```python
from build123d import *

# Parameters (mm, degrees)
F0_DEPTH     = 70
F1_W         = 75
F1_H         = 15
F4_DEPTH     = 2
F2_T1_DEPTH  = 11
F2_T3_DEPTH  = 73
F2_T5_DEPTH  = 67
F2_T7_DEPTH  = 71
F2_S11_W     = 2.04
F2_S11_H     = 2.04
F2_T12_DEPTH = 2.04
F2_S17_W     = 2.04
F2_S17_H     = 2.04
F2_T18_DEPTH = 2.04
F2_S23_W     = 2.04
F2_S23_H     = 2.04
F2_T24_DEPTH = 2.04
F2_S29_W     = 2.04
F2_S29_H     = 2.04
F2_T30_DEPTH = 2.04
F2_T37_DEPTH = 73
F2_T42_DEPTH = 72
F2_T50_DEPTH = 72
F2_T55_DEPTH = 73
F2_T62_DEPTH = 16
F2_T67_DEPTH = 16


# Not quite as in the source:
# - a fillet or chamfer that OpenCascade refuses, or shapes differently, is made with other operations: its cross-section is extruded or revolved along the edge and cut away or added
# - a feature names something its author has since deleted; it is built from what else it names


with BuildPart() as f0:
    # F3 (on Top) → F0 (new body)
    with BuildSketch(Plane.XY):
        Polygon((-37.5, 15), (-37.5, 0), (37.5, 0), (37.5, 15), (33.5, 15), (33.5, 13), (35.5, 13), (35.5, 2), (-35.5, 2), (-35.5, 13), (-33.5, 13), (-33.5, 15), align=None)
    extrude(amount=F0_DEPTH)

    # F1 (on face) → F4 (join)
    with BuildSketch(Plane(origin=(0, 0, 0), x_dir=(1, 0, 0), z_dir=(0, 0, -1))):
        with Locations((0, -7.5)):
            Rectangle(F1_W, F1_H)
    extrude(amount=-F4_DEPTH)

    # F2: fillet of radius 2 on 13 edges, made by hand

    # F2_s2 → F2_t1 (cut)
    with BuildSketch(Plane.XZ.offset(-13)):
        with BuildLine():
            ThreePointArc((37.5, 2), (36.9142135624, 0.5857864376), (35.5, 0))
            Line((35.5, 0), (37.5, 0))
            Line((37.5, 0), (37.5, 2))
        make_face()
        with BuildLine():
            ThreePointArc((-37.5, 2), (-36.9142135624, 0.5857864376), (-35.5, 0))
            Line((-35.5, 0), (-37.5, 0))
            Line((-37.5, 0), (-37.5, 2))
        make_face()
    extrude(amount=F2_T1_DEPTH, mode=Mode.SUBTRACT)

    # F2_s4 → F2_t3 (cut)
    with BuildSketch(Plane.XY.offset(2)):
        with BuildLine():
            ThreePointArc((-37.5, 2), (-36.9142135624, 0.5857864376), (-35.5, 0))
            Line((-35.5, 0), (-37.5, 0))
            Line((-37.5, 0), (-37.5, 2))
        make_face()
        with BuildLine():
            ThreePointArc((35.5, 0), (36.9142135624, 0.5857864376), (37.5, 2))
            Line((37.5, 2), (37.5, 0))
            Line((37.5, 0), (35.5, 0))
        make_face()
        with BuildLine():
            ThreePointArc((-37.5, 13), (-36.9142135624, 14.4142135624), (-35.5, 15))
            Line((-35.5, 15), (-37.5, 15))
            Line((-37.5, 15), (-37.5, 13))
        make_face()
        with BuildLine():
            ThreePointArc((37.5, 13), (36.9142135624, 14.4142135624), (35.5, 15))
            Line((35.5, 15), (37.5, 15))
            Line((37.5, 15), (37.5, 13))
        make_face()
        with BuildLine():
            ThreePointArc((-33.5, 13), (-34.0857864376, 14.4142135624), (-35.5, 15))
            Line((-35.5, 15), (-33.5, 15))
            Line((-33.5, 15), (-33.5, 13))
        make_face()
        with BuildLine():
            ThreePointArc((33.5, 13), (34.0857864376, 14.4142135624), (35.5, 15))
            Line((35.5, 15), (33.5, 15))
            Line((33.5, 15), (33.5, 13))
        make_face()
    extrude(amount=F2_T3_DEPTH, mode=Mode.SUBTRACT)

    # F2_s6 → F2_t5 (cut)
    with BuildSketch(Plane.YZ.offset(-33.5)):
        with BuildLine():
            ThreePointArc((13, 2), (14.4142135624, 1.4142135624), (15, 0))
            Line((15, 0), (15, 2))
            Line((15, 2), (13, 2))
        make_face()
    extrude(amount=F2_T5_DEPTH, mode=Mode.SUBTRACT)

    # F2_s8 → F2_t7 (cut)
    with BuildSketch(Plane.YZ.offset(-35.5)):
        with BuildLine():
            ThreePointArc((0, 2), (0.5857864376, 0.5857864376), (2, 0))
            Line((2, 0), (0, 0))
            Line((0, 0), (0, 2))
        make_face()
        with BuildLine():
            ThreePointArc((15, 2), (14.4142135624, 0.5857864376), (13, 0))
            Line((13, 0), (15, 0))
            Line((15, 0), (15, 2))
        make_face()
    extrude(amount=F2_T7_DEPTH, mode=Mode.SUBTRACT)


with BuildPart() as f2_tool10:
    # F2_s11 → F2_t12 (new body)
    with BuildSketch(Plane.XZ.offset(-2)):
        with Locations((36.52, 0.98)):
            Rectangle(F2_S11_W, F2_S11_H)
    extrude(amount=F2_T12_DEPTH)

    # F2_s13 → F2_t14 (revolve, cut)
    with BuildSketch(Plane(origin=(35.5, 2, 2), x_dir=(-0.7071067812, 0, 0.7071067812), z_dir=(0.7071067812, 0, 0.7071067812))):
        with BuildLine():
            ThreePointArc((0, -2), (2, 0), (0, 2))
            Line((0, 2), (0, -2))
        make_face()
    revolve(axis=Axis((35.5, 2, 2), (0, -1, 0)), mode=Mode.SUBTRACT)


with BuildPart() as f0_1:
    add(f0.part)

    # F2_t9: cut F2_tool10
    add(f2_tool10.part, mode=Mode.SUBTRACT)


with BuildPart() as f2_tool16:
    # F2_s17 → F2_t18 (new body)
    with BuildSketch(Plane.YZ.offset(35.5)):
        with Locations((14.02, 0.98)):
            Rectangle(F2_S17_W, F2_S17_H)
    extrude(amount=F2_T18_DEPTH)

    # F2_s19 → F2_t20 (revolve, cut)
    with BuildSketch(Plane(origin=(35.5, 13, 2), x_dir=(0, -0.7071067812, 0.7071067812), z_dir=(0, 0.7071067812, 0.7071067812))):
        with BuildLine():
            ThreePointArc((0, -2), (2, 0), (0, 2))
            Line((0, 2), (0, -2))
        make_face()
    revolve(axis=Axis((35.5, 13, 2), (1, 0, 0)), mode=Mode.SUBTRACT)


with BuildPart() as f0_2:
    add(f0_1.part)

    # F2_t15: cut F2_tool16
    add(f2_tool16.part, mode=Mode.SUBTRACT)


with BuildPart() as f2_tool22:
    # F2_s23 → F2_t24 (new body)
    with BuildSketch(Plane.YZ.offset(-35.5)):
        with Locations((14.02, 0.98)):
            Rectangle(F2_S23_W, F2_S23_H)
    extrude(amount=-F2_T24_DEPTH)

    # F2_s25 → F2_t26 (revolve, cut)
    with BuildSketch(Plane(origin=(-35.5, 13, 2), x_dir=(0, -0.7071067812, 0.7071067812), z_dir=(0, -0.7071067812, -0.7071067812))):
        with BuildLine():
            ThreePointArc((0, -2), (2, 0), (0, 2))
            Line((0, 2), (0, -2))
        make_face()
    revolve(axis=Axis((-35.5, 13, 2), (-1, 0, 0)), mode=Mode.SUBTRACT)


with BuildPart() as f0_3:
    add(f0_2.part)

    # F2_t21: cut F2_tool22
    add(f2_tool22.part, mode=Mode.SUBTRACT)


with BuildPart() as f2_tool28:
    # F2_s29 → F2_t30 (new body)
    with BuildSketch(Plane.YZ.offset(-35.5)):
        with Locations((0.98, 0.98)):
            Rectangle(F2_S29_W, F2_S29_H)
    extrude(amount=-F2_T30_DEPTH)

    # F2_s31 → F2_t32 (revolve, cut)
    with BuildSketch(Plane(origin=(-35.5, 2, 2), x_dir=(0, 0.7071067812, 0.7071067812), z_dir=(0, -0.7071067812, 0.7071067812))):
        with BuildLine():
            ThreePointArc((0, -2), (2, 0), (0, 2))
            Line((0, 2), (0, -2))
        make_face()
    revolve(axis=Axis((-35.5, 2, 2), (-1, 0, 0)), mode=Mode.SUBTRACT)


with BuildPart() as f0_4:
    add(f0_3.part)

    # F2_t27: cut F2_tool28
    add(f2_tool28.part, mode=Mode.SUBTRACT)


with BuildPart() as f2_tool35:
    # F2_s36 → F2_t37 (new body)
    with BuildSketch(Plane.XY.offset(-3)):
        with BuildLine():
            ThreePointArc((-33.5, 13), (-34.0857864376, 14.4142135624), (-35.5, 15))
            Line((-35.5, 15), (-33.5, 15))
            Line((-33.5, 15), (-33.5, 13))
        make_face()
    extrude(amount=F2_T37_DEPTH)

    split(bisect_by=Plane.XY.offset(2), keep=Keep.BOTTOM)

    split(bisect_by=Plane.XY, keep=Keep.TOP)


with BuildPart() as f2_tool40:
    # F2_s41 → F2_t42 (new body)
    with BuildSketch(Plane.YZ.offset(-38.5)):
        with BuildLine():
            ThreePointArc((13, 2), (14.4142135624, 1.4142135624), (15, 0))
            Line((15, 0), (15, 2))
            Line((15, 2), (13, 2))
        make_face()
    extrude(amount=F2_T42_DEPTH)

    split(bisect_by=Plane.YZ.offset(-33.5), keep=Keep.BOTTOM)

    split(bisect_by=Plane.YZ.offset(-35.5), keep=Keep.TOP)


with BuildPart() as f2_tool35_1:
    add(f2_tool35.part)

    # F2_t45: intersect F2_tool40
    add(f2_tool40.part, mode=Mode.INTERSECT)


with BuildPart() as f0_5:
    add(f0_4.part)

    # F2_t33: cut F2_tool35
    add(f2_tool35_1.part, mode=Mode.SUBTRACT)


with BuildPart() as f2_tool48:
    # F2_s49 → F2_t50 (new body)
    with BuildSketch(Plane.YZ.offset(-33.5)):
        with BuildLine():
            ThreePointArc((13, 2), (14.4142135624, 1.4142135624), (15, 0))
            Line((15, 0), (15, 2))
            Line((15, 2), (13, 2))
        make_face()
    extrude(amount=F2_T50_DEPTH)

    split(bisect_by=Plane.YZ.offset(35.5), keep=Keep.BOTTOM)

    split(bisect_by=Plane.YZ.offset(33.5), keep=Keep.TOP)


with BuildPart() as f2_tool53:
    # F2_s54 → F2_t55 (new body)
    with BuildSketch(Plane.XY.offset(-3)):
        with BuildLine():
            ThreePointArc((33.5, 13), (34.0857864376, 14.4142135624), (35.5, 15))
            Line((35.5, 15), (33.5, 15))
            Line((33.5, 15), (33.5, 13))
        make_face()
    extrude(amount=F2_T55_DEPTH)

    split(bisect_by=Plane.XY.offset(2), keep=Keep.BOTTOM)

    split(bisect_by=Plane.XY, keep=Keep.TOP)


with BuildPart() as f2_tool48_1:
    add(f2_tool48.part)

    # F2_t58: intersect F2_tool53
    add(f2_tool53.part, mode=Mode.INTERSECT)


with BuildPart() as f0_6:
    add(f0_5.part)

    # F2_t46: cut F2_tool48
    add(f2_tool48_1.part, mode=Mode.SUBTRACT)


with BuildPart() as f2_tool60:
    # F2_s61 → F2_t62 (new body)
    with BuildSketch(Plane.XZ.offset(3)):
        with BuildLine():
            ThreePointArc((35.5, 4), (34.9142135624, 2.5857864376), (33.5, 2))
            Line((33.5, 2), (35.5, 2))
            Line((35.5, 2), (35.5, 4))
        make_face()
    extrude(amount=-F2_T62_DEPTH)

    split(bisect_by=Plane.XZ, keep=Keep.BOTTOM)


with BuildPart() as f0_7:
    add(f0_6.part)

    # F2_t59: union F2_tool60
    add(f2_tool60.part)


with BuildPart() as f2_tool65:
    # F2_s66 → F2_t67 (new body)
    with BuildSketch(Plane.XZ.offset(-13)):
        with BuildLine():
            ThreePointArc((-35.5, 4), (-34.9142135624, 2.5857864376), (-33.5, 2))
            Line((-33.5, 2), (-35.5, 2))
            Line((-35.5, 2), (-35.5, 4))
        make_face()
    extrude(amount=F2_T67_DEPTH)

    split(bisect_by=Plane.XZ, keep=Keep.BOTTOM)


with BuildPart() as f0_8:
    add(f0_7.part)

    # F2_t64: union F2_tool65
    add(f2_tool65.part)


solid = f0_8.part
```
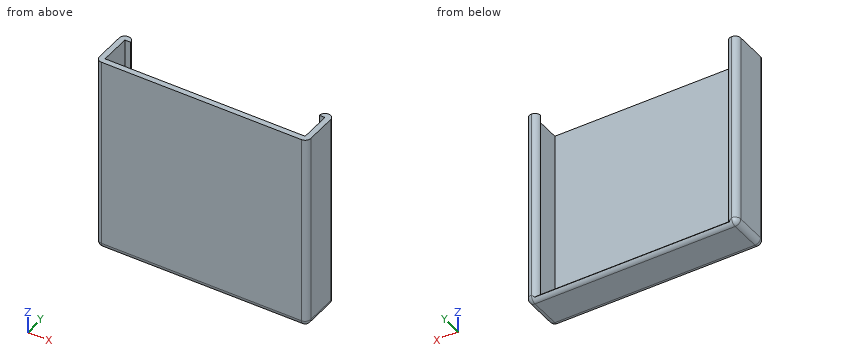
Design review of the part built by this model. Coordinates are the model's own, in mm. Coordinates: 2 decimals unless noted, no trailing zeros. Loops run counter-clockwise (first coordinate to the right, second up) from the corner with the lowest first, then second, coordinate; pieces in that order, holes last. Notation, with made-up numbers: (36, 29.5) - (88, 29.5) arc R13 cw to (88, 34.5) - close; hole circle Ø8 at (60, -10). An arc over 180 degrees is marked (long way). Use CSV: the item, a comma, the result in double quotes. Start each with the question number.
1) Wall thickness on L1, parallel to X at y = 3.25, z = 30; L2, parallel to Y at x = 16.5, z = 14: over which ranges is each line inside the solid? List them lowest first. Write a range as from..to.
2) Consider section A-A on y = 10. Write out the cut boundary in (x, z).
3) Consider section C-C on z = 31. Write out the cut boundary in (x, y), then the cut area to 3 significant figures.
4) Consider section B-B on x = 26. Write out the cut boundary in (y, z), then the cut area to 3 significant figures.
5) For pin 1 Ø8 at (x, y) = (11.5, 11) entering from +Z, flat-tipped, find the tip position at first contact; note if it passes through.
Geometry says:
1,L1,"-37.5..-35.5, 35.5..37.5"
1,L2,"0..2"
2,outline,"(-37.5, 2) arc R2 ccw to (-35.5, 0) - (35.5, 0) arc R2 ccw to (37.5, 2) - (37.5, 70) - (35.5, 70) - (35.5, 4) arc R2 cw to (33.5, 2) - (-33.5, 2) arc R2 cw to (-35.5, 4) - (-35.5, 70) - (-37.5, 70) - close"
3,outline,"(-37.5, 2) arc R2 ccw to (-35.5, 0) - (35.5, 0) arc R2 ccw to (37.5, 2) - (37.5, 13) arc R2 ccw to (33.5, 13) - (35.5, 13) - (35.5, 2) - (-35.5, 2) - (-35.5, 13) - (-33.5, 13) arc R2 ccw to (-37.5, 13) - close"
3,area,"205 mm^2"
4,outline,"(0, 2) arc R2 ccw to (2, 0) - (13, 0) arc R2 ccw to (14.73, 1) arc R2 ccw to (13, 2) - (2, 2) - (2, 70) - (0, 70) - close"
4,area,"164 mm^2"
5,pin 1,"z = 2"
